Autodesk Inventor part; units mm, degrees
ref_plane "YZ Plane" through (0, 0, 0) normal (1, 0, 0) x (0, 1, 0)
ref_plane "XZ Plane" through (0, 0, 0) normal (0, 1, 0) x (-1, 0, 0)
ref_plane "XY Plane" through (0, 0, 0) normal (0, 0, 1) x (1, 0, 0)
sketch "スケッチ1" plane through (0, 0, 0) normal (0, 0, 1) x (1, 0, 0)
  line L0 (0, 0) -> (11, 0)
  line L1 (11, 0) -> (11, 12)
  line L2 (11, 12) -> (0, 12)
  line L3 (0, 12) -> (0, 0)
  dimension "d0" = 11
  dimension "d1" = 12
extrude "押し出し1" add sketch "スケッチ1" along normal blind 2.1
sketch "スケッチ2" plane through (0, 0, 2.1) normal (0, 0, 1) x (1, 0, 0)
  circle A0 centre (5.5, 6.5) radius 2
  line L0 (0, 12) -> (0, 0)
  line L1 (11, 12) -> (0, 12)
  line L2 (3.7679, 7.5) -> (7.2321, 7.5)
  dimension "d4" = 4
  dimension "d5" = 5.5
  dimension "d6" = 5.5
  dimension "d7" = 3
extrude "押し出し2" cut sketch "スケッチ2" against normal through all contours A0 L2 picked at (5.5553, 6.2487)
sketch "スケッチ3" plane through (0, 0, 2.1) normal (0, 0, 1) x (1, 0, 0)
  line L0 (0, 12) -> (0, 0)
  line L1 (0, 9) -> (3, 12)
  line L2 (11, 12) -> (0, 12)
  line L3 (0, 1) -> (1, 0)
  line L4 (0, 0) -> (11, 0)
  line L5 (5.5, 12) -> (5.5, 0)
  line L6 (11, 9) -> (8, 12)
  line L7 (11, 1) -> (10, 0)
  dimension "d10" = 45
  dimension "d12" = 1
  dimension "d13" = 3
  dimension "d14" = 1
extrude "押し出し3" cut sketch "スケッチ3" against normal through all contours L2 L1 L0
sketch "スケッチ4" plane through (0, 0, 2.1) normal (0, 0, 1) x (1, 0, 0)
  line L0 (11, 12) -> (3, 12)
  line L1 (8, 12) -> (11, 9)
  line L2 (11, 0) -> (11, 12)
  point P0 (0, 0)
  dimension "d17" = 3
  dimension "d18" = 3
extrude "押し出し4" cut sketch "スケッチ4" against normal through all
sketch "スケッチ5" plane through (0, 0, 2.1) normal (0, 0, 1) x (1, 0, 0)
  line L0 (0, 9) -> (0, 0)
  line L1 (0, 1.25) -> (1.25, 0)
  line L2 (0, 0) -> (11, 0)
  dimension "d21" = 1.25
  dimension "d29" = 1.25
extrude "押し出し5" cut sketch "スケッチ5" against normal through all
sketch "スケッチ6" plane through (0, 0, 2.1) normal (0, 0, 1) x (1, 0, 0)
  line L0 (11, 0) -> (11, 9)
  line L1 (11, 1.25) -> (9.75, 0)
  line L2 (1.25, 0) -> (11, 0)
  point P0 (0, 0)
  dimension "d25" = 1.25
  dimension "d26" = 1.25
extrude "押し出し6" cut sketch "スケッチ6" against normal through all
sketch "スケッチ7" plane through (1.25, 0, 0) normal (0, -1, 0) x (1, 0, 0)
  point P0 (-1.25, 0)
sketch "スケッチ8" plane through (0, 0, 2.1) normal (0, 0, 1) x (1, 0, 0)
  point P0 (0, 0)
sketch "スケッチ9" plane through (0, 0, 2.1) normal (0, 0, 1) x (1, 0, 0)
  point P0 (0, 0)
sketch "スケッチ10" plane through (1.25, 0, 0) normal (0, -1, 0) x (1, 0, 0)
  line L0 (3.75, 0.2) -> (4.75, 0.2)
  line L1 (4.75, 0.2) -> (4.75, 0)
  line L2 (4.75, 0) -> (3.75, 0)
  line L3 (3.75, 0) -> (3.75, 0.2)
  line L4 (0, 0) -> (8.5, 0)
  line L5 (6.25, 0.2) -> (7.25, 0.2)
  line L6 (7.25, 0.2) -> (7.25, 0)
  line L7 (7.25, 0) -> (6.25, 0)
  line L8 (6.25, 0) -> (6.25, 0.2)
  line L9 (9.75, 2.1) -> (9.75, 0)
  point P0 (-1.25, 0)
  dimension "d31" = 1
  dimension "d36" = 0.2
  dimension "d37" = 1
  dimension "d38" = 2.5
sketch "スケッチ12" plane through (1.25, 0, 0) normal (0, -1, 0) x (1, 0, 0)
  line L0 (6.25, 2.1) -> (6.25, 0)
  line L1 (6.75, 0) -> (9.75, 0)
  line L2 (6.25, 0.2) -> (7.25, 0.2)
  line L3 (7.25, 0.2) -> (7.25, 0)
  line L4 (7.25, 0) -> (6.25, 0)
  line L5 (6.25, 0) -> (6.25, 0.2)
  point P0 (-1.25, 0)
  dimension "d34" = 1
  dimension "d35" = 0.2
extrude "押し出し7" add sketch "スケッチ10" along normal blind 1.4 contours L0 L1 L2 L3
extrude "押し出し8" add sketch "スケッチ12" along normal blind 1.4
sketch "スケッチ13" plane through (1.25, 0, 0) normal (0, -1, 0) x (1, 0, 0)
  line L0 (6.25, 0) -> (2.25, 0)
  line L1 (2.25, 0.2) -> (1.25, 0.2)
  line L2 (1.25, 0.2) -> (1.25, 0)
  line L3 (1.25, 0) -> (2.25, 0)
  line L4 (2.25, 0) -> (2.25, 0.2)
  line L5 (-1.25, 0) -> (-1.25, 2.1)
  point P0 (2.5179, 0)
  point P1 (5.9821, 0)
  dimension "d43" = 0.2
  dimension "d44" = 1
  dimension "d45" = 2.5
extrude "押し出し9" add sketch "スケッチ13" along normal blind 1.4
sketch "スケッチ14" plane through (3, 12, 2.1) normal (0, 1, 0) x (1, 0, 0)
  line L0 (2, 1.9) -> (3, 1.9)
  line L1 (0.5, 2.1) -> (4.5, 2.1)
  line L2 (2, 1.9) -> (3, 1.9)
  line L3 (3, 1.9) -> (3, 2.1)
  line L4 (3, 2.1) -> (2, 2.1)
  line L5 (2, 2.1) -> (2, 1.9)
  point P0 (-3, 2.1)
  point P1 (0.7679, 2.1)
  point P2 (4.2321, 2.1)
  dimension "d48" = 1
extrude "押し出し10" add sketch "スケッチ14" along normal blind 1.5
properties part number "3SR08_ポテンショメータ"
Design review of the part built by this model. Coordinates are the model's own, in mm. A direction names the side the tool comes from. Coordinates: 2 decimals unless noted, no trailing zeros. Write each loop counter-clockwise with the first axis right and the second up, starting at its lowest first coordinate (ties: lowest second). Pieces come first, ordered by that corner, then holes.
1) Insertion check: pin 1 (0.8 mm diameter, centred on x = 5.5, y = 13, fed in from +Z); pin 2 (0.6 mm diameter, centred on x = 6, z = 1, fed in from -Y); pin 3 (0.6 mm diameter, centred on x = 5, z = 1.5, fed in from +Y). Each pin has a flat end and moves straight along its axis. Give the tip position at first contact, or say it passes through.
2) To check wall thickness, follow L1, parallel to X at y = 6.5, z = 1.25; L2, parallel to Y at x = 5.5, z = 0.55; L3, parallel to X at y = 6, z = 1.15. State the ranges of each line that lie inside material, in increasing order.
3) Mouldability with a two-part tool opening along X and no side actions: class faces 4 (the flat face through (5.5, 12.7, 0.2)), 5 (the cylindrical face through (5.44, 4.5, 1.06)), 6 (the flat face through (9, 11, 1)) as +X half, -X half, draft (parallel to the pull), parting line (faces both ways), or undercut.
4) Add section B-B (y = 6.5). Write out the cut boundary in (x, z), plus the area to 3 significant figures.
5) Add section D-D (x = 1). Write out the cut boundary in (y, z), plus the area to 3 significant figures.
6) Add section C-C (z = 1.5). Write out the cut boundary in (x, y), plus the area to 3 significant figures.
7) Machinability: for faces 1 (the flat face through (5, 7.5, 1)), 2 (the flat face through (11, 5, 1)), 3 (the flat face through (3, -1, 0.2)), which of the approach directions +Z, -Z, +X, -X, +Y, -Y give a long, thin tool a straight path to every point of the face, cutting with its end or side? Answer none if there is none.
8) Add section A-A (x = 5.5). Write out the cut boundary in (y, z).
Check result:
1. pin 1: stops at z = 0.2
1. pin 2: stops at y = 0
1. pin 3: stops at y = 12
2. L1: x = 0 to 3.5, 7.5 to 11
2. L2: y = 0 to 4.5, 7.5 to 12
2. L3: x = 0 to 3.56, 7.44 to 11
3. face 4: draft
3. face 5: undercut
3. face 6: +X half
4. outline: (0, 0) - (3.5, 0) - (3.5, 2.1) - (0, 2.1) - close; (7.5, 0) - (11, 0) - (11, 2.1) - (7.5, 2.1) - close
4. area: 14.7 mm2
5. outline: (0.25, 0) - (10, 0) - (10, 2.1) - (0.25, 2.1) - close
5. area: 20.5 mm2
6. outline: (0, 1.25) - (1.25, 0) - (9.75, 0) - (11, 1.25) - (11, 9) - (8, 12) - (3, 12) - (0, 9) - close; hole (3.77, 7.5) arc R2 ccw (long way) to (7.23, 7.5) - close
6. area: 111 mm2
7. face 1: +Z, -Z
7. face 2: +Z, -Z, +X, +Y, -Y
7. face 3: +Z, +X, -X, -Y
8. outline: (-1.4, 0) - (4.5, 0) - (4.5, 2.1) - (0, 2.1) - (0, 0.2) - (-1.4, 0.2) - close; (7.5, 0) - (13.5, 0) - (13.5, 0.2) - (12, 0.2) - (12, 2.1) - (7.5, 2.1) - close
